Geometry: final body of the model. Coordinates: model frame, mm. Face numbers are marked on the shaded views. A direction names the side the tool comes from. Coordinates: 2 decimals unless noted, no trailing zeros. Write each loop counter-clockwise with the first axis right and the second up, starting at its lowest first coordinate (ties: lowest second). Pieces come first, ordered by that corner, then holes. Notation, with made-up numbers: (80, 6) - (116, 6) arc R22 ccw to (116, 27) - close; hole circle Ø6 at (32.5, -39.5). An arc over 180 degrees is marked (long way). Put each result on its own line as item: value.
```python
from build123d import *

# Parameters (mm, degrees)
F0_R     = 17.8
F1_DEPTH = 12.5
F2_R     = 11
F3_DEPTH = 25
F4_R     = 14
F5_DEPTH = 6
F6_R     = 13.8
F7_DEPTH = 2.2


with BuildPart() as f1:
    # F0 (on Top) → F1 (new body)
    with BuildSketch(Plane.XY):
        Circle(F0_R)
    extrude(amount=F1_DEPTH)

    # F2 (on face) → F3 (cut)
    with BuildSketch(Plane.XY.offset(12.5)):
        Circle(F2_R)
    extrude(amount=-F3_DEPTH, mode=Mode.SUBTRACT)

    # F4 (on face) → F5 (cut)
    with BuildSketch(Plane(origin=(0, 0, 0), x_dir=(1, 0, 0), z_dir=(0, 0, -1))):
        Circle(F4_R)
    extrude(amount=-F5_DEPTH, mode=Mode.SUBTRACT)

    # F6 (on face) → F7 (cut)
    with BuildSketch(Plane.XY.offset(12.5)):
        Circle(F6_R)
    extrude(amount=-F7_DEPTH, mode=Mode.SUBTRACT)


solid = f1.part
```
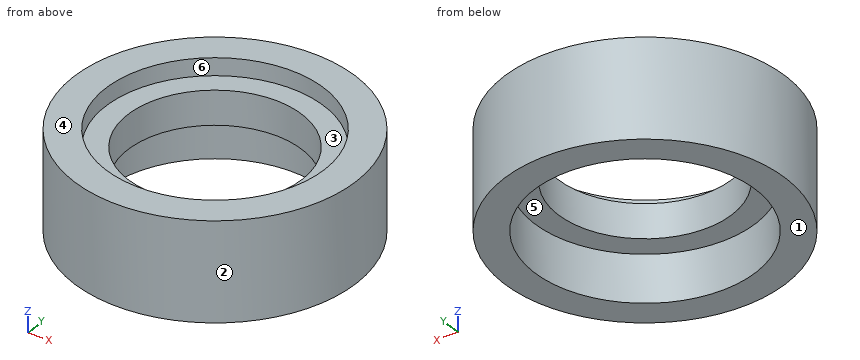
1. Ray query, probe 1 along Y at (x, z) = (0, 7.75); probe 2 along Y at (x, z) = (-0.5, 5.5); probe 3 along Z at (x, y) = (-13, 2). Return the intervals inside material, ascending. Write a range as from..to.
Answer below:
probe 1: y = -17.8..-11, 11..17.8
probe 2: y = -17.79..-13.99, 13.99..17.79
probe 3: z = 6..10.3
2. Set-up query: the marked faces 4, 5 and 6. Return all of +Z, -Z, +X, -X, +Y, -Y with unobstructed straight access to the full face (end or side cutting, diameter ignored); none if empty.
Answer below:
face 4: +Z, +X, -X, +Y, -Y
face 5: -Z
face 6: +Z
3. Section query B-B (y = -9). Return loops of the section in (x, z).
Answer below:
outline: (-15.36, 0) - (-10.72, 0) - (-10.72, 6) - (-6.32, 6) - (-6.32, 10.3) - (-10.46, 10.3) - (-10.46, 12.5) - (-15.36, 12.5) - close; (6.32, 6) - (10.72, 6) - (10.72, 0) - (15.36, 0) - (15.36, 12.5) - (10.46, 12.5) - (10.46, 10.3) - (6.32, 10.3) - close
4. Pin query (flat end, axial travel): pin 1 Ø5 at (x, z) = (-12, 3) entering from -Y; pin 2 Ø6 at (y, z) = (-3.5, 10) entering from +X; pin 3 Ø1.5 at (x, z) = (-14, 6.5) entering from +Y. Return the tip coordinate at first contact, or that it passes through.
Answer below:
pin 1: stops at y = -15.05
pin 2: stops at x = 17.79
pin 3: stops at y = 11.89
5. Mould query, pull axis X, two halves, no side actions, for the marked faces 1, 2 and 3. Classes: +X half, -X half, draft (parallel to the pull), parting line (faces both ways), or undercut.
Answer below:
face 1: draft
face 2: parting line
face 3: undercut
6. Section query A-A (x = 0). Return loops of the section in (y, z).
Answer below:
outline: (-17.8, 0) - (-14, 0) - (-14, 6) - (-11, 6) - (-11, 10.3) - (-13.8, 10.3) - (-13.8, 12.5) - (-17.8, 12.5) - close; (11, 6) - (14, 6) - (14, 0) - (17.8, 0) - (17.8, 12.5) - (13.8, 12.5) - (13.8, 10.3) - (11, 10.3) - close
7. Section query D-D (y = -15.5). Return loops of the section in (x, z).
Answer below:
outline: (-8.75, 0) - (8.75, 0) - (8.75, 12.5) - (-8.75, 12.5) - close
8. Section query C-C (z = 2). Return loops of the section in (x, y).
Answer below:
outline: circle Ø35.6 at (0, 0); hole circle Ø28 at (0, 0)
